from build123d import *

# Parameters (mm, degrees)
SKETCH1_W           = 54
SKETCH1_H           = 38
BOSS_EXTRUDE1_DEPTH = 3
SKETCH2_W           = 5
SKETCH2_H           = 5
SKETCH2_R           = 1.6
BOSS_EXTRUDE2_DEPTH = 16


with BuildPart() as part:
    # Sketch1 → Boss-Extrude1 (new body)
    with BuildSketch(Plane.XY):
        with Locations((27, 19)):
            Rectangle(SKETCH1_W, SKETCH1_H)
    extrude(amount=BOSS_EXTRUDE1_DEPTH)

    # Sketch2 → Boss-Extrude2 (add)
    # profile 1 of 2: a face of its own
    with BuildSketch(Plane.XY):
        with Locations((12.9, 7.7)):
            Rectangle(SKETCH2_W, SKETCH2_H)
        with Locations((12.9, 7.7)):
            Circle(SKETCH2_R, mode=Mode.SUBTRACT)
    # profile 2 of 2: a face of its own
    with BuildSketch(Plane.XY):
        with Locations((51.5, 15.29)):
            Rectangle(SKETCH2_W, SKETCH2_H)
        with Locations((51.5, 15.29)):
            Circle(SKETCH2_R, mode=Mode.SUBTRACT)
    extrude(amount=-BOSS_EXTRUDE2_DEPTH)


solid = part.part
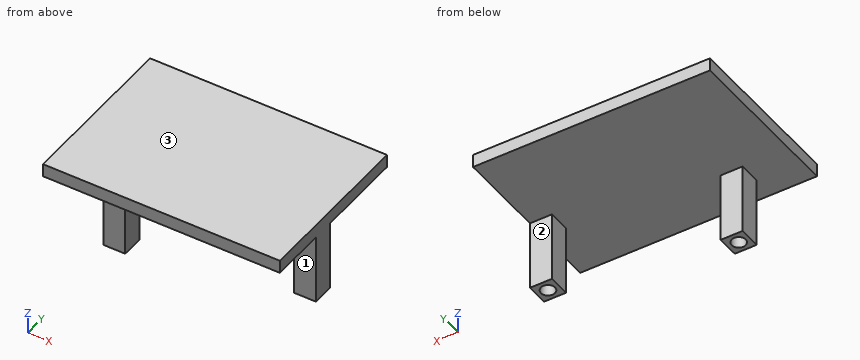
Could you check a few things on this model? Use its own coordinates, in mm. Face numbers are marked on the shaded views. A direction names the side the tool comes from. Coordinates: 2 decimals unless noted, no trailing zeros. Order: outer loops, then holes, each group sorted by start corner. A loop starts at its lowest first (then second) coordinate and runs counter-clockwise, first axis right, second up. Notation, with made-up numbers: (45, 51.5) - (59, 51.5) arc R13 cw to (59, 67.5) - close; hole circle Ø9 at (57.25, -10). An arc over 180 degrees is marked (long way). Answer in a Markdown table with one row per item. Add a question column.
(1) I need wall thicknesses on L1, parallel to Y at x = 12.9, z = -8; L2, parallel to Z at x = 4, y = 22.5; L3, parallel to X at y = 8, z = -11.25. Which ranges of each line are inside material? Lowest first, please.
(2) If we section it at A-A, the plane z = -8.5: Please give me the cut outline in (x, y), then the cut area to 3 significant figures.
(3) If we section it at B-B, the plane y = 7.7: Please give me the cut outline in (x, z).
(4) If we section it at D-D, the plane x = 42.5: Please give me the cut outline in (y, z), then the cut area to 3 significant figures.
(5) On a 3-axis mill with a long thin cutter (end or side, diameter ignored), from which of +Z, -Z, +X, -X, +Y, -Y can I reach the whole of each face in a straight line? I mean the marked faces 1, 2 and 3. Say none if no direction works.
(6) If we section it at C-C, the plane x = 51.5: Please give me the cut outline in (y, z), then the cut area to 3 significant figures.
(7) Will these pins go through, and if not, where does the flat tip stop? pin 1 (2 mm diameter, centred on y = 5.5, z = -5.5, fed in from -X); pin 2 (6 mm diameter, centred on x = 35.5, y = 8.5, fed in from -Z); pin 3 (1.5 mm diameter, centred on y = 16, z = -5.5, fed in from -X).
Results are:
| question | item | result |
|---|---|---|
| 1 | L1 | y = 5.2 to 6.1, 9.3 to 10.2 |
| 1 | L2 | z = 0 to 3 |
| 1 | L3 | x = 10.4 to 11.33, 14.47 to 15.4 |
| 2 | outline | (10.4, 5.2) - (15.4, 5.2) - (15.4, 10.2) - (10.4, 10.2) - close; (49, 12.79) - (54, 12.79) - (54, 17.79) - (49, 17.79) - close; hole circle Ø3.2 at (12.9, 7.7); hole circle Ø3.2 at (51.5, 15.29) |
| 2 | area | 33.9 mm2 |
| 3 | outline | (0, 0) - (10.4, 0) - (10.4, -16) - (11.3, -16) - (11.3, 0) - (14.5, 0) - (14.5, -16) - (15.4, -16) - (15.4, 0) - (54, 0) - (54, 3) - (0, 3) - close |
| 4 | outline | (0, 0) - (38, 0) - (38, 3) - (0, 3) - close |
| 4 | area | 114 mm2 |
| 5 | face 1 | -Z, +X, -X, -Y |
| 5 | face 2 | -Z, +X, -X, +Y |
| 5 | face 3 | +Z, +X, -X, +Y, -Y |
| 6 | outline | (0, 0) - (12.79, 0) - (12.79, -16) - (13.69, -16) - (13.69, 0) - (16.89, 0) - (16.89, -16) - (17.79, -16) - (17.79, 0) - (38, 0) - (38, 3) - (0, 3) - close |
| 6 | area | 143 mm2 |
| 7 | pin 1 | stops at x = 10.4 |
| 7 | pin 2 | stops at z = 0 |
| 7 | pin 3 | stops at x = 49 |
